Geometry: see drawing. Coordinates: mm, zero at the bounding-box minimum. Give positions to 0.01 mm unless a question says otherwise; leave off trailing zeros. Loops run counter-clockwise (first coordinate to the right, second up) from the corner with the lowest first, then second, coordinate; pieces in that order, holes last. Notation, with made-up numbers: M -1,-18.75 L 56,-18.75 A4 cw 56,-12.75 Z; hole C -6.75,28.25 d11. An arc over 180 degrees is marked long. Answer in a Markdown table with one row per item.
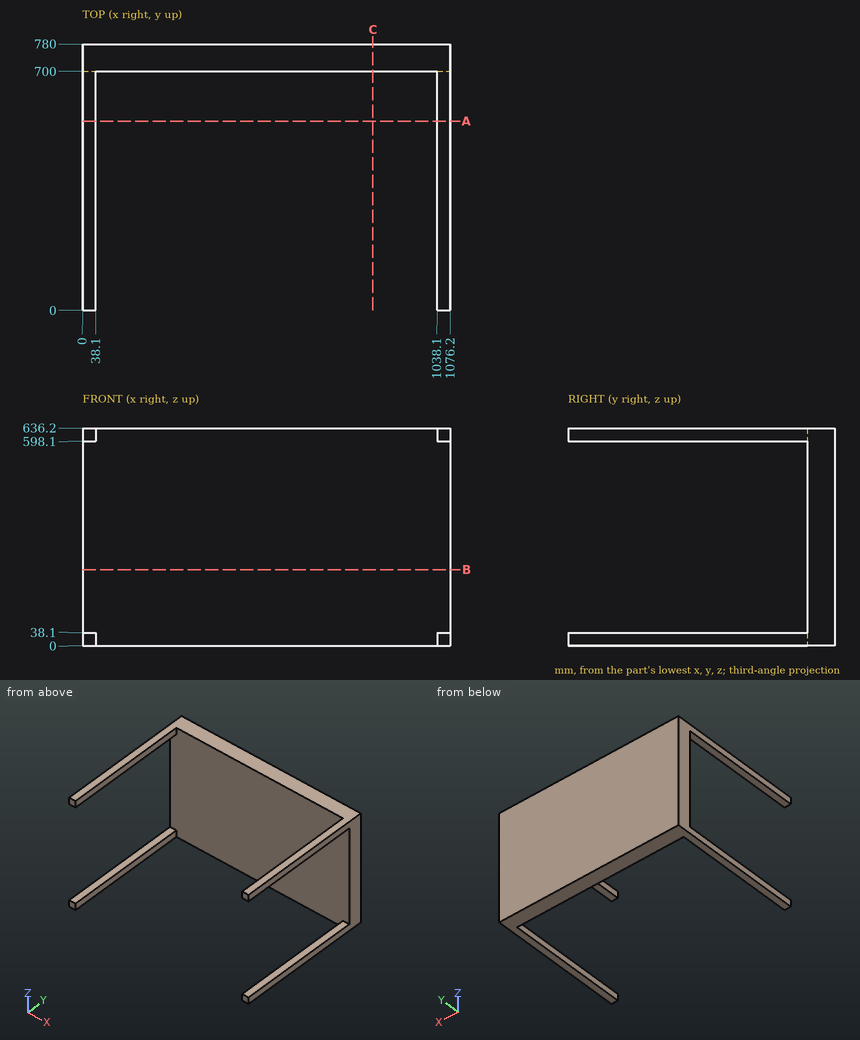
1) Section B-B, the plane z = 222.5. Return loops of the section in (x, y), then the cut area to 3 significant figures.
Reply:
| item | result |
|---|---|
| outline | M 0,700 L 1076.2,700 L 1076.2,780 L 0,780 Z |
| area | 86,100 mm² |
2) Section C-C, the plane x = 850.5. Return loops of the section in (y, z).
Reply:
| item | result |
|---|---|
| outline | M 700,0 L 780,0 L 780,636.2 L 700,636.2 Z |
3) Material intervals for L1, parallel to Y at x = 214, z = 558.5, sorted ascending.
Reply:
| item | result |
|---|---|
| L1 | y = 700 to 780 |
4) Pin query (flat end, axial travel): pin 1 Ø2 at (x, z) = (180.5, 240.5) entering from -Y. Return the tip coordinate at first contact, or that it passes through.
Reply:
| item | result |
|---|---|
| pin 1 | stops at y = 700 |
5) Section A-A, the plane y = 554.5. Return loops of the section in (x, z).
Reply:
| item | result |
|---|---|
| outline | M 0,0 L 38.1,0 L 38.1,38.1 L 0,38.1 Z; M 0,598.1 L 38.1,598.1 L 38.1,636.2 L 0,636.2 Z; M 1038.1,0 L 1076.2,0 L 1076.2,38.1 L 1038.1,38.1 Z; M 1038.1,598.1 L 1076.2,598.1 L 1076.2,636.2 L 1038.1,636.2 Z |
